Here's how the part is built. I have some questions about the finished solid (model axes, mm). Face numbers are marked on the shaded views. A direction names the side the tool comes from. Coordinates: 2 decimals unless noted, no trailing zeros. Write each loop counter-clockwise with the first axis right and the second up, starting at its lowest first coordinate (ties: lowest second). Pieces come first, ordered by that corner, then holes. Notation, with made-up numbers: (66, 87) -> (83, 87) arc R26 ccw to (83, 123) -> close; hole circle Ø5 at (10, 37.25). An arc over 180 degrees is marked (long way). Put each result on its own line as item: value. Start each with the question number.
Item 1: I want a section at D-D, the plane x = 51.5. List the corners of the cut face in (y, z) for me, then the cut area to 3 significant figures.
Item 2: I want a section at B-B, the plane z = 12. List the corners of the cut face in (x, y) for me.
Item 3: For pin 1 (5 mm diameter, centred on y = -8, z = 9.5, fed in from -X); pin 2 (12 mm diameter, centred on x = 22.5, y = 4, fed in from +Z); pin 3 (4 mm diameter, centred on x = 84, y = 9.5, fed in from +Z), each with a flat end and sliding along its axis, tell me the tip position at first contact or that it passes through.
Item 4: I want a section at C-C, the plane z = 45. List the corners of the cut face in (x, y) for me, then the cut area to 3 significant figures.
Item 5: I need wall thicknesses on line 1 (Y direction, x = 0, z = 5); line 2 (X direction, y = -3, z = 5); line 3 (X direction, y = 22.5, z = 28.5). Which ranges of each line are inside material? Lowest first, please. Write a range as [from, to].
Item 6: On a 3-axis mill with a long thin cutter (end or side, diameter ignored), from which of +Z, -Z, +X, -X, +Y, -Y can I reach the whole of each face in a straight line? I mean the marked faces 1, 2, 3, 4 and 5. Say none if no direction works.
Item 7: If we mould it in two halves opening along X, with no side actions, what happens to the marked faces 6, 7 and 8? For each: released by +X, released by -X, zero draft, split by the parting line, or undercut.
Item 8: I want a section at A-A, the plane y = 0. List the corners of the cut face in (x, z) for me.
from build123d import *

# Parameters (mm, degrees)
F0_R     = 6.35
F1_DEPTH = 20
F2_DEPTH = 30
F3_DEPTH = 55
F5_DEPTH = 90.001
F7_DEPTH = 60.001


with BuildPart() as f1:
    # F0 (on Top) → F1 (new body)
    with BuildSketch(Plane.XY):
        with BuildLine():
            Line((20, -15), (20, 15))
            Line((20, 15), (0, 15))
            ThreePointArc((0, 15), (-15, 0), (0, -15))
            Line((0, -15), (20, -15))
        make_face()
        Circle(F0_R, mode=Mode.SUBTRACT)
    extrude(amount=F1_DEPTH)

    # F0 (on Top) → F2 (join)
    with BuildSketch(Plane.XY):
        Polygon((110, 30), (55, 30), (55, -30), (110, -30), (110, -15), (85, -15), (85, 15), (110, 15), align=None)
        Polygon((55, 30), (20, 30), (20, 15), (20, -15), (20, -30), (55, -30), align=None)
    extrude(amount=F2_DEPTH)

    # F0 (on Top) → F3 (join)
    with BuildSketch(Plane.XY):
        Polygon((55, 30), (20, 30), (20, 15), (20, -15), (20, -30), (55, -30), align=None)
    extrude(amount=F3_DEPTH)

    # F4 (on face) → F5 (cut, through all)
    with BuildSketch(Plane(origin=(20, 0, 0), x_dir=(0, -1, 0), z_dir=(-1, 0, 0))):
        with BuildLine():
            Line((20, 55), (-20, 55))
            ThreePointArc((-20, 55), (0, 35), (20, 55))
        make_face()
    extrude(amount=-F5_DEPTH, mode=Mode.SUBTRACT)

    # F6 (on face) → F7 (cut, through all)
    with BuildSketch(Plane.XZ.offset(30)):
        Polygon((49.226497, 10), (55, 0), (75, 0), (80.773503, 10), align=None)
    extrude(amount=-F7_DEPTH, mode=Mode.SUBTRACT)


solid = f1.part
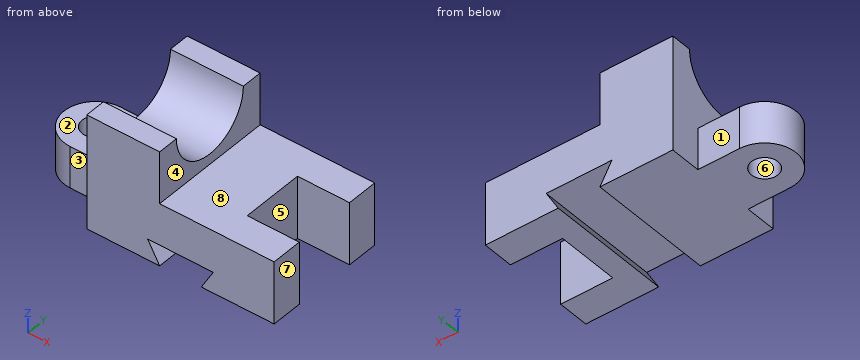
Calculated:
1. outline: (-30, 0) -> (30, 0) -> (30, 6.06) -> (-30, 6.06) -> close; (-30, 10) -> (30, 10) -> (30, 55) -> (20, 55) arc R20 cw to (-20, 55) -> (-30, 55) -> close
1. area: 2,440 mm2
2. outline: (0, -15) -> (20, -15) -> (20, -30) -> (110, -30) -> (110, -15) -> (85, -15) -> (85, 15) -> (110, 15) -> (110, 30) -> (20, 30) -> (20, 15) -> (0, 15) arc R15 ccw to start; hole circle Ø12.7 at (0, 0)
3. pin 1: stops at x = -13.96
3. pin 2: stops at z = 37.68
3. pin 3: stops at z = 30
4. outline: (20, -30) -> (55, -30) -> (55, -17.32) -> (20, -17.32) -> close; (20, 17.32) -> (55, 17.32) -> (55, 30) -> (20, 30) -> close
4. area: 888 mm2
5. line 1: y = [-15, -6.35], [6.35, 15]
5. line 2: x = [-14.7, -5.6], [5.6, 52.11], [77.89, 85]
5. line 3: x = [20, 110]
6. face 1: +Z, -Z, -X, +Y
6. face 2: +Z, -X, +Y, -Y
6. face 3: +Z, -Z, -X, -Y
6. face 4: +Z, +X, +Y, -Y
6. face 5: +Z, -Z, +X
7. face 6: undercut
7. face 7: released by +X
7. face 8: zero draft
8. outline: (-15, 0) -> (-6.35, 0) -> (-6.35, 20) -> (-15, 20) -> close; (6.35, 0) -> (55, 0) -> (49.23, 10) -> (80.77, 10) -> (75, 0) -> (85, 0) -> (85, 30) -> (55, 30) -> (55, 35) -> (20, 35) -> (20, 20) -> (6.35, 20) -> close
